Can you work these out from the model? Positions are in its coordinate system, mm. A direction names the side the tool comes from. Give positions to 0.01 mm unless a question says otherwise; leave off trailing zeros. Order: outer loops, then holes, each group sorted by start corner. A loop starts at its lowest first (then second) coordinate and runs counter-clockwise, first axis right, second up.
Item 1: I want a section at A-A, the plane x = 0. Write out the boundary of the cut face in (y, z).
Item 2: I want a section at C-C, the plane y = -0.75. Write out the boundary of the cut face in (x, z).
Item 3: Which directions (+Z, -Z, +X, -X, +Y, -Y) give clear straight access to the entire face, cutting with the end or side of a thin tool? Please do faces 1 (the flat face through (1.421, 1, -2)), 2 (the flat face through (-4.34, 1.48, 27.3)), 3 (the cylindrical face through (0.82, -2.17, -16.32)).
Item 4: I want a section at D-D, the plane z = -17. Write out the boundary of the cut face in (x, y).
Item 5: I'm going to push flat-ended pins straight in: pin 1 Ø2 at (x, y) = (-2.5, -1.5) entering from +Z; pin 2 Ø0.9 at (x, z) = (0, -2) entering from -Y; pin 3 Ø2 at (y, z) = (1, -1.5) entering from -X; pin 4 Ø1 at (y, z) = (-1.5, 7) entering from +X. Where does each tip first touch, or does it pass through?
Item 6: If we mould it in two halves opening along X, with no side actions, what happens to faces 4 (the flat face through (-3.537, 1, 15)), 5 (the flat face through (7.598, 1, 12)), 6 (the flat face through (-5, 0, 11)), 7 (the flat face through (0, 1, 5))? For each: +X half, -X half, draft (parallel to the pull), parting line (faces both ways), or undercut.
Item 7: I want a section at B-B, the plane z = 2.5. Write out the boundary of the cut face in (x, y), then the cut area to 3 significant figures.
Item 8: If I drill on line 1 along Z through (x, y) = (-1.5, 1); line 2 along Y through (x, z) = (-1.5, 2.5); line 3 along Z through (x, y) = (-1.75, 3.5), over which ranges is the centre line in solid material (lowest first)?
```python
from build123d import *

# Parameters (mm, degrees)
BOSS_EXTRUDE1_DEPTH = 3
SKETCH2_W           = 2.84238377
SKETCH2_H           = 2.456975153
BOSS_EXTRUDE2_DEPTH = 4
SKETCH3_R           = 3.785280903
BOSS_EXTRUDE3_DEPTH = 25


with BuildPart() as part:
    # Sketch1 → Boss-Extrude1 (new body)
    with BuildSketch(Plane(origin=(0, 0, 0), x_dir=(1, 0, 0), z_dir=(0, 1, 0))):
        Polygon((-7.401746725, 0), (7.598253275, 0), (7.598253275, -25), (6.222707424, -28.945414847), (4.317186999, -25), (4.317186999, -5), (-3.537117904, -5), (-3.537117904, -25), (-5.163870247, -29.665938865), (-7.401746725, -25), align=None)
    extrude(amount=BOSS_EXTRUDE1_DEPTH)

    # Sketch2 → Boss-Extrude2 (add)
    with BuildSketch(Plane(origin=(0, 0, 0), x_dir=(-1, 0, 0), z_dir=(0, 0, -1))):
        with Locations((0, 1.475753534)):
            Rectangle(SKETCH2_W, SKETCH2_H)
    extrude(amount=BOSS_EXTRUDE2_DEPTH)

    # Sketch3 → Boss-Extrude3 (add)
    with BuildSketch(Plane(origin=(0, 0, -4), x_dir=(-1, 0, 0), z_dir=(0, 0, -1))):
        with Locations((0, 1.524246465)):
            Circle(SKETCH3_R)
    extrude(amount=BOSS_EXTRUDE3_DEPTH)


solid = part.part
```
Results list:
1. outline: (-2.26, -29) - (5.31, -29) - (5.31, -4) - (2.7, -4) - (2.7, 0) - (3, 0) - (3, 5) - (0, 5) - (0, 0) - (0.25, 0) - (0.25, -4) - (-2.26, -4) - close
2. outline: (-3.03, -29) - (3.03, -29) - (3.03, -4) - (-3.03, -4) - close
3. face 1: +X, +Y, -Y
3. face 2: +Z, +Y, -Y
3. face 3: -Z
4. outline: circle Ø7.57 at (0, 1.52)
5. pin 1: stops at z = -4
5. pin 2: stops at y = 0.25
5. pin 3: stops at x = -1.42
5. pin 4: passes through
6. face 4: undercut
6. face 5: +X half
6. face 6: draft
6. face 7: undercut
7. outline: (-7.4, 0) - (7.6, 0) - (7.6, 3) - (-7.4, 3) - close
7. area: 45.0 mm2
8. line 1: z = -29 to -4, 0 to 5
8. line 2: y = 0 to 3
8. line 3: z = -29 to -4
